For this review, take the finished solid that the model builds, in its own axes (mm). A direction names the side the tool comes from. Coordinates: 2 decimals unless noted, no trailing zeros. Loops run counter-clockwise (first coordinate to the right, second up) from the corner with the lowest first, then second, coordinate; pieces in that order, holes last.
1. Clearance check with flat-ended pins moving along their axes: P1, Ø2, axis at y = 0.5, z = -82, coming from the -X side; P2, Ø2.5, axis at x = 166.5, y = 1.5, coming from the -Z side; P3, Ø2, axis at x = 165, y = 0.5, coming from the +Z side. State where each tip first meets the part, or that it passes through.
2. Mouldability with a two-part tool opening along Z and no side actions: class faces 1 (the face through (136.4, 2, -72)), 2 (the face through (101, 2, 0)), 3 (the face through (158.87, 2.46, -66.14)), 4 (the face through (5, 3, -90)) as pulls with the +Z half, pulls with the -Z half, needs draft (parallel to the pull), parting line crosses it, or undercut.
3. Machinability: for faces 5 (the face through (28, 3, -5)), 6 (the face through (200, 3, -28.5)), 7 (the face through (125.6, 2, -72)), which of the approach directions +Z, -Z, +X, -X, +Y, -Y give a long, thin tool a straight path to every point of the face, cutting with its end or side? Answer none if there is none.
4. Take a section at B-B, the plane y = 2.95. Count the separate pieces of the cut face and the enclosed holes in it, then the cut area to 3 significant figures.
5. Take a section at A-A, the plane x = 131. State the section outline as (y, z) points.
6. Take a section at C-C, the plane z = -88.5. State the section outline as (x, y) points.
7. To check wall thickness, follow probe 1 along Z at (x, y) = (184.5, 1.9); probe 2 along X at (y, z) = (1.5, -35); probe 3 along Z at (x, y) = (101.5, 3.75). State the ranges of each line that lie inside material, in increasing order.
```python
from build123d import *

# Parameters (mm, degrees)
SKETCH1_W            = 203
SKETCH1_H            = 107
BOSS_EXTRUDE1_DEPTH  = 5
SKETCH3_W            = 51
SKETCH3_H            = 5
CUT_EXTRUDE1_DEPTH   = 230.527776097
SKETCH4_W            = 5
SKETCH4_H            = 28.5
CUT_EXTRUDE2_DEPTH   = 230.527776097
CUT_EXTRUDE3_DEPTH   = 230.527776097
SKETCH10_R           = 3.25
CUT_EXTRUDE4_DEPTH   = 230.527776097
M3_CLEARANCE_HOLE1_D = 3.4
SKETCH13_W           = 9
SKETCH13_H           = 12
CUT_EXTRUDE5_DEPTH   = 230.527776097
M3_CLEARANCE_HOLE2_D = 3.4
M3_CLEARANCE_HOLE3_D = 3.4


with BuildPart() as part:
    # Sketch1 → Boss-Extrude1 (new body)
    with BuildSketch(Plane(origin=(0, 0, 0), x_dir=(1, 0, 0), z_dir=(0, 1, 0))):
        with Locations((101.5, 53.5)):
            Rectangle(SKETCH1_W, SKETCH1_H)
    extrude(amount=BOSS_EXTRUDE1_DEPTH)

    # Sketch3 → Cut-Extrude1 (cut, through all)
    with BuildSketch(Plane(origin=(0, 5, 0), x_dir=(1, 0, 0), z_dir=(0, 1, 0))):
        with Locations((25.5, 104.5)):
            Rectangle(SKETCH3_W, SKETCH3_H)
        with Locations((177.5, 104.5)):
            Rectangle(SKETCH3_W, SKETCH3_H)
        with Locations((25.5, 2.5)):
            Rectangle(SKETCH3_W, SKETCH3_H)
        with Locations((177.5, 2.5)):
            Rectangle(SKETCH3_W, SKETCH3_H)
    extrude(amount=-CUT_EXTRUDE1_DEPTH, mode=Mode.SUBTRACT)

    # Sketch4 → Cut-Extrude2 (cut, through all)
    with BuildSketch(Plane(origin=(0, 5, 0), x_dir=(1, 0, 0), z_dir=(0, 1, 0))):
        with Locations((2.5, 92.75)):
            Rectangle(SKETCH4_W, SKETCH4_H)
        with Locations((2.5, 14.25)):
            Rectangle(SKETCH4_W, SKETCH4_H)
        with Locations((200.5, 14.25)):
            Rectangle(SKETCH4_W, SKETCH4_H)
        with Locations((200.5, 92.75)):
            Rectangle(SKETCH4_W, SKETCH4_H)
    extrude(amount=-CUT_EXTRUDE2_DEPTH, mode=Mode.SUBTRACT)

    # Sketch7 → Cut-Extrude3 (cut, through all)
    with BuildSketch(Plane.XZ):
        with BuildLine():
            Line((164.385100742, -69.683506307), (164.385100742, -74.945459))
            ThreePointArc((164.385100742, -74.945459), (158.96865866, -78.137919554), (153.585100742, -74.890312225))
            Line((153.585100742, -74.890312225), (153.585100742, -69.754043843))
            ThreePointArc((153.585100742, -69.754043843), (158.961713268, -66.137919554), (164.385100742, -69.683506307))
        make_face()
        with BuildLine():
            Line((136.4, -69.402295461), (136.4, -74.632878398))
            ThreePointArc((136.4, -74.632878398), (131, -78.007665824), (125.6, -74.632878398))
            Line((125.6, -74.632878398), (125.6, -69.402295461))
            ThreePointArc((125.6, -69.402295461), (131, -66.007665824), (136.4, -69.402295461))
        make_face()
    extrude(amount=-CUT_EXTRUDE3_DEPTH, mode=Mode.SUBTRACT)

    # Sketch10 → Cut-Extrude4 (cut, through all)
    with BuildSketch(Plane.XZ):
        with Locations(Location((131, -35, 0), (0, 0, 270))):
            Circle(SKETCH10_R)
    extrude(amount=-CUT_EXTRUDE4_DEPTH, mode=Mode.SUBTRACT)

    # M3 Clearance Hole1 (through all)
    with Locations(Plane(origin=(0, 0, 0), x_dir=(-1, 0, 0), z_dir=(0, -1, 0))):
        with Locations((-18.5, 14.6), (-184.5, 14.6), (-184.5, 92.4), (-18.5, 92.4)):
            Hole(M3_CLEARANCE_HOLE1_D / 2)

    # Sketch13 → Cut-Extrude5 (cut, through all)
    with BuildSketch(Plane(origin=(0, 0, 0), x_dir=(-1, 0, 0), z_dir=(0, -1, 0))):
        with Locations((-159, 35)):
            Rectangle(SKETCH13_W, SKETCH13_H)
    extrude(amount=-CUT_EXTRUDE5_DEPTH, mode=Mode.SUBTRACT)

    # M3 Clearance Hole2 (through all)
    with Locations(Plane(origin=(0, 0, 0), x_dir=(-1, 0, 0), z_dir=(0, -1, 0))):
        with Locations((-150.95, 35), (-167.05, 35)):
            Hole(M3_CLEARANCE_HOLE2_D / 2)

    # M3 Clearance Hole3 (through all)
    with Locations(Plane(origin=(0, 0, 0), x_dir=(-1, 0, 0), z_dir=(0, -1, 0))):
        with Locations((-101.5, 104.5), (-101.5, 2.5)):
            Hole(M3_CLEARANCE_HOLE3_D / 2)


solid = part.part
```
Results list:
1. P1: stops at x = 5
1. P2: stops at z = -102
1. P3: stops at z = -5
2. face 1: undercut
2. face 2: pulls with the +Z half
2. face 3: undercut
2. face 4: needs draft
3. face 5: +Z, -X, +Y, -Y
3. face 6: +Z, +X, +Y, -Y
3. face 7: +Y, -Y
4. separate pieces: 1
4. enclosed holes: 12
4. area: 19,800 mm2
5. outline: (0, -107) - (5, -107) - (5, -78.01) - (0, -78.01) - close; (0, -66.01) - (5, -66.01) - (5, -38.25) - (0, -38.25) - close; (0, -31.75) - (5, -31.75) - (5, 0) - (0, 0) - close
6. outline: (5, 0) - (198, 0) - (198, 5) - (5, 5) - close
7. probe 1: z = -102 to -94.1, -90.7 to -16.3, -12.9 to -5
7. probe 2: x = 0 to 127.75, 134.25 to 149.25, 152.65 to 154.5, 163.5 to 165.35, 168.75 to 203
7. probe 3: z = -107 to -106.2, -102.8 to -4.2, -0.8 to 0
